Source: three-view drawing plus pictorial views. Frame: mm from the lowest corner of the part. Round coordinates to 2 decimals unless told otherwise and drop trailing zeros. Loops run counter-clockwise (first coordinate to the right, second up) from the corner with the lowest first, then second, coordinate; pieces in that order, holes last. Notation, with made-up numbers: (-17, 76.5) -> (-13, 76.5) arc R18 cw to (-13, 88.5) -> close; hole circle Ø1 at (6.5, -27). An arc over 180 degrees is marked (long way). One line per question, with ' | ' between items. Start each with the question number.
Q1. Cut plane D-D on z = 56.5. Return loops of the section in (x, y).
Q2. Contact query for flat-ended pins moving along their axis: P1, Ø2, axis at y = 45.5, z = 8.5, coming from the -X side (1 decimal); P2, Ø2, axis at x = 51.5, z = 29.5, coming from the +Y side (1 decimal); P3, Ø8, axis at x = 46, z = 53, coming from the +Y side. Output: stop coordinate, or through.
Q3. Cut plane A-A on z = 29.5. Return loops of the section in (x, y).
Q4. Cut plane C-C on x = 5. Return loops of the section in (y, z).
Q5. Material intervals for L1, parallel to Y at x = 9.5, z = 40 (1 decimal); L2, parallel to Y at x = 54, z = 13 (1 decimal); L3, parallel to X at y = 12.5, z = 19.5, sorted ascending.
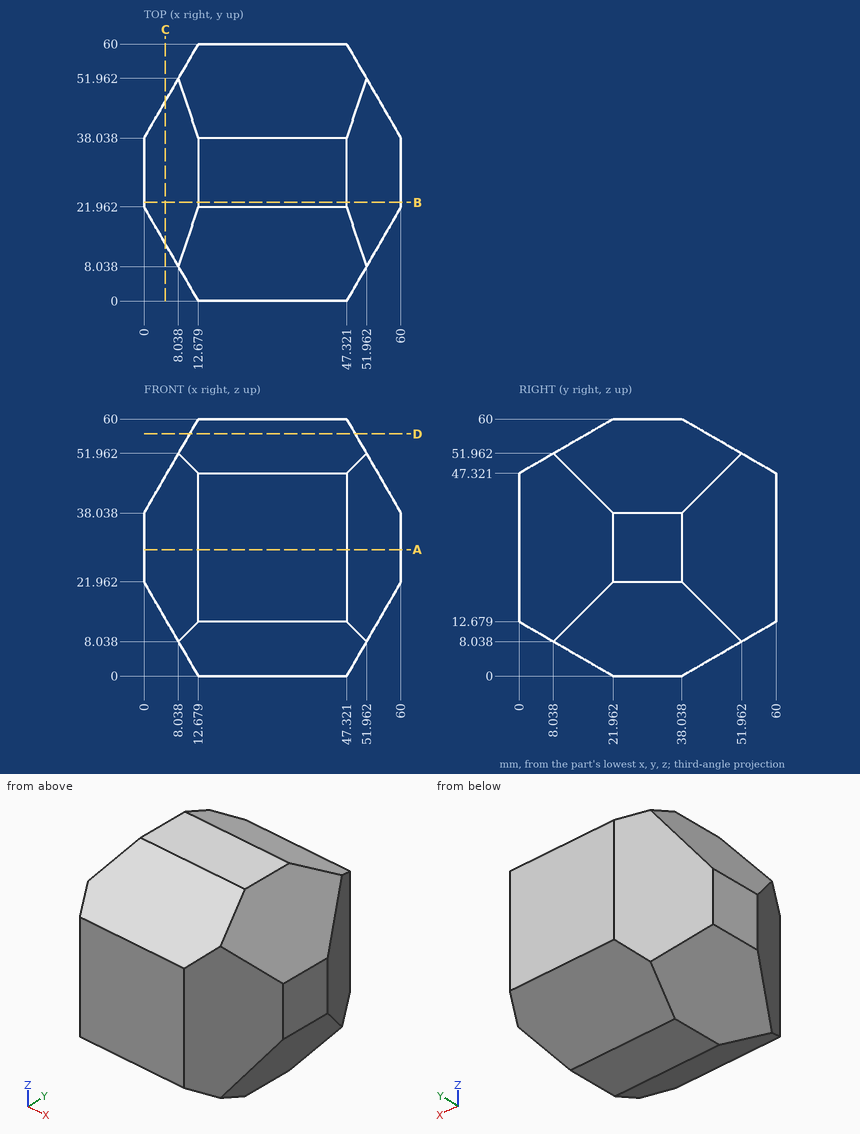
Results:
1) outline: (10.66, 15.9) -> (49.34, 15.9) -> (49.34, 44.1) -> (10.66, 44.1) -> close
2) P1: x = 7.2 | P2: y = 54.5 | P3: y = 57.09
3) outline: (0, 21.96) -> (12.68, 0) -> (47.32, 0) -> (60, 21.96) -> (60, 38.04) -> (47.32, 60) -> (12.68, 60) -> (0, 38.04) -> close
4) outline: (13.3, 13.3) -> (46.7, 13.3) -> (46.7, 46.7) -> (13.3, 46.7) -> close
5) L1: 5.5 to 54.5 | L2: 11.6 to 48.4 | L3: 5.46 to 54.54
